Verification items for the finished model (mm, model axes). A direction names the side the tool comes from. Coordinates: 2 decimals unless noted, no trailing zeros. Loops run counter-clockwise (first coordinate to the right, second up) from the corner with the lowest first, then second, coordinate; pieces in that order, holes last. Notation, with made-up numbers: (84, 16) - (121, 16) arc R20 ccw to (121, 46) - close; hole circle Ø6 at (8, 74). An arc over 180 degrees is marked (long way). One line per item, written item: value. Start each with the question number.
(1) Section check A-A (x = 35). Record the boundary of the cut face in (y, z), plus the area to 3 significant figures.
(2) Draft check along Z on faces 5 (the face through (40.8, -5.7, -30.8)), 6 (the face through (-30.8, -5.7, -40.8)), 7 (the face through (-5, -5.7, 40.8)). Enter one of: +Z half, -Z half, draft (parallel to the pull), parting line (faces both ways), or undercut.
(3) Section check C-C (y = -5). Record the boundary of the cut face in (x, z).
(4) Set-up check for faces 1 (the face through (-40.5, -5.74, 5.15)), 2 (the face through (40.5, -5.7, 30.2)), 3 (the face through (30.8, -5.7, 40.8)), 4 (the face through (30.2, -5.7, -40.5)): record each of +Z, -Z, +X, -X, +Y, -Y from which the full face is reachable in a straight line by a thin tool's end or side.
(5) Gauge pin test, flat end, axial feed: P1, Ø2, axis at y = -6, z = 9.5, coming from the -X side. Record the tip position at first contact, or that the pin passes through.
(6) Thickness scan on probe 1 along X at (y, z) = (-6.95, -36.5); probe 2 along Z at (x, y) = (-46, -4.2); probe 3 along X at (y, z) = (-4.85, 42.5). Record the ranges inside material, lowest first. Write a range as [from, to].
(7) Section check D-D (z = -20). Record the boundary of the cut face in (x, y).
(8) Section check B-B (z = -34.5). Record the boundary of the cut face in (x, y), plus the area to 3 significant figures.
```python
from build123d import *

# Parameters (mm, degrees)
F0_W     = 101.6
F0_H     = 101.6
F1_DEPTH = 7.62
F3_DEPTH = 3.81


with BuildPart() as f1:
    # F0 (on Front) → F1 (new body)
    with BuildSketch(Plane.XZ):
        Rectangle(F0_W, F0_H)
    extrude(amount=F1_DEPTH)

    # F2 (on face) → F3 (intersect)
    with BuildSketch(Plane.XZ.offset(7.62)):
        Polygon((-16.9333333333, 16.9333333333), (-10.16, 30.48), (-50.8, 50.8), (-30.48, 10.16), align=None)
        Polygon((10.16, 30.48), (0, 50.8), (-10.16, 30.48), (0, 25.4), align=None)
        Polygon((0, 25.4), (-10.16, 30.48), (-16.9333333333, 16.9333333333), align=None)
        Polygon((16.9333333333, 16.9333333333), (10.16, 30.48), (0, 25.4), align=None)
        Polygon((50.8, 50.8), (10.16, 30.48), (16.9333333333, 16.9333333333), (30.48, 10.16), align=None)
        Polygon((50.8, 0), (30.48, 10.16), (25.4, 0), (30.48, -10.16), align=None)
        Polygon((50.8, -50.8), (30.48, -10.16), (16.9333333333, -16.9333333333), (10.16, -30.48), align=None)
        Polygon((-10.16, -30.48), (0, -50.8), (10.16, -30.48), (0, -25.4), align=None)
        Polygon((-16.9333333333, -16.9333333333), (-30.48, -10.16), (-50.8, -50.8), (-10.16, -30.48), align=None)
        Polygon((-25.4, 0), (-30.48, 10.16), (-50.8, 0), (-30.48, -10.16), align=None)
        Polygon((-25.4, 0), (-16.9333333333, 16.9333333333), (-30.48, 10.16), align=None)
        Polygon((0, 25.4), (-16.9333333333, 16.9333333333), (-25.4, 0), (-16.9333333333, -16.9333333333), (0, -25.4), (16.9333333333, -16.9333333333), (25.4, 0), (16.9333333333, 16.9333333333), align=None)
        Polygon((10.16, -30.48), (16.9333333333, -16.9333333333), (0, -25.4), align=None)
        Polygon((30.48, -10.16), (25.4, 0), (16.9333333333, -16.9333333333), align=None)
        Polygon((30.48, 10.16), (16.9333333333, 16.9333333333), (25.4, 0), align=None)
        Polygon((-16.9333333333, -16.9333333333), (-25.4, 0), (-30.48, -10.16), align=None)
        Polygon((0, -25.4), (-16.9333333333, -16.9333333333), (-10.16, -30.48), align=None)
    extrude(amount=-F3_DEPTH, mode=Mode.INTERSECT)


solid = f1.part
```
Responses:
1. outline: (-7.62, -42.9) - (-3.81, -42.9) - (-3.81, -19.2) - (-7.62, -19.2) - close; (-7.62, -7.9) - (-3.81, -7.9) - (-3.81, 7.9) - (-7.62, 7.9) - close; (-7.62, 19.2) - (-3.81, 19.2) - (-3.81, 42.9) - (-7.62, 42.9) - close
1. area: 241 mm²
2. face 5: undercut
2. face 6: -Z half
2. face 7: +Z half
3. outline: (-50.8, -50.8) - (-10.16, -30.48) - (0, -50.8) - (10.16, -30.48) - (50.8, -50.8) - (30.48, -10.16) - (50.8, 0) - (30.48, 10.16) - (50.8, 50.8) - (10.16, 30.48) - (0, 50.8) - (-10.16, 30.48) - (-50.8, 50.8) - (-30.48, 10.16) - (-50.8, 0) - (-30.48, -10.16) - close
4. face 1: -X, +Y, -Y
4. face 2: +X, +Y, -Y
4. face 3: +Z, +Y, -Y
4. face 4: -Z, +Y, -Y
5. P1: stops at x = -33.8
6. probe 1: x = [-43.65, -22.2], [-7.15, 7.15], [22.2, 43.65]
6. probe 2: z = [-48.4, -41.2], [-2.4, 2.4], [41.2, 48.4]
6. probe 3: x = [-46.65, -34.2], [-4.15, 4.15], [34.2, 46.65]
7. outline: (-35.4, -7.62) - (35.4, -7.62) - (35.4, -3.81) - (-35.4, -3.81) - close
8. outline: (-42.65, -7.62) - (-18.2, -7.62) - (-18.2, -3.81) - (-42.65, -3.81) - close; (-8.15, -7.62) - (8.15, -7.62) - (8.15, -3.81) - (-8.15, -3.81) - close; (18.2, -7.62) - (42.65, -7.62) - (42.65, -3.81) - (18.2, -3.81) - close
8. area: 248 mm²
